Design review of the part built by this model. Coordinates are the model's own, in mm. Face numbers are marked on the shaded views. A direction names the side the tool comes from. Round coordinates to 2 decimals unless told otherwise and drop trailing zeros. Loops run counter-clockwise (first coordinate to the right, second up) from the corner with the lowest first, then second, coordinate; pieces in that order, holes last. Notation, with made-up numbers: (45, -39) - (93, -39) arc R22 cw to (93, -5) - close; hole circle Ø3 at (36.25, -19.5). An arc over 180 degrees is marked (long way). Return JSON: item names as keys, results as strings. Group by question number.
(1) We need section B-B, the plane z = 6.35. Write out the cut boundary in (x, y) (1 decimal), and give its area (3 significant figures).
(2) The part is to be moulded in two halves that separate along Y. For the marked faces 1, 2 and 3, say which applies: pulls with the +Y half, pulls with the -Y half, needs draft (parallel to the pull), parting line crosses it, or undercut.
(3) Clearance check with flat-ended pins moving along their axes: pin 1 (9 mm diameter, centred on x = 26.67, z = 6.35, fed in from -Y) (3 decimals); pin 2 (3 mm diameter, centred on x = 21, y = 0.5, fed in from -Z); pin 3 (10 mm diameter, centred on y = 11, z = 3, fed in from -X); pin 4 (12.5 mm diameter, centred on x = 32.5, y = 11, fed in from +Z). State where each tip first meets the part, or that it passes through.
(4) For the marked faces 4 and 5, list the 3-axis set-ups (+Z, -Z, +X, -X, +Y, -Y) from which the entire face can be reached by the end or side of a thin tool; tool diameter is ignored.
(5) We need section D-D, the plane y = 4.5. Write out the cut boundary in (x, z), and give its area (3 significant figures).
(6) Wall thickness on L1, parallel to X at y = -2.4, z = 6.35; L2, parallel to Y at x = 31, z = 4.5 (1 decimal); L3, parallel to X at y = -5, z = 6.35: over which ranges is each line inside the solid? List them lowest first. Write a range as [from, to].
(7) We need section A-A, the plane x = 26.67. Give the number of separate pieces and of enclosed holes in the cut face, and give its area (3 significant figures).
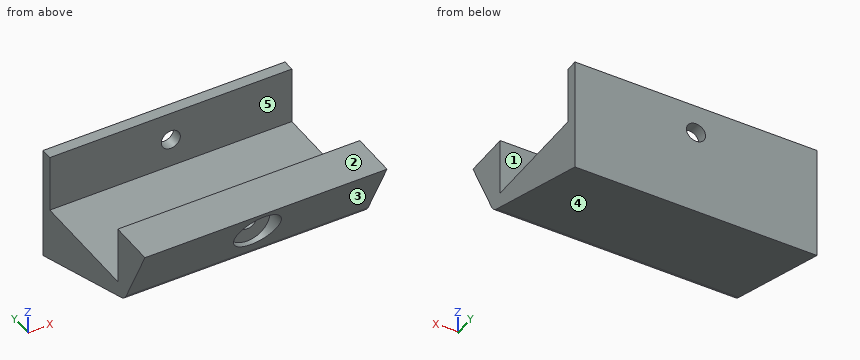
Autodesk Inventor part; units mm, degrees
ref_plane "YZ Plane" through (0, 0, 0) normal (1, 0, 0) x (0, 1, 0)
ref_plane "XZ Plane" through (0, 0, 0) normal (0, 1, 0) x (-1, 0, 0)
ref_plane "XY Plane" through (0, 0, 0) normal (0, 0, 1) x (1, 0, 0)
sketch "Sketch1" plane through (0, 0, 0) normal (1, 0, 0) x (0, 1, 0)
  line L0 (0, 0) -> (25.4, 0)
  line L1 (25.4, 0) -> (25.4, 12.7)
  line L2 (0, 0) -> (0, 12.7)
  line L3 (25.4, 12.7) -> (27.9305, 12.7)
  line L4 (27.9305, 12.7) -> (27.9305, 0)
  line L5 (0, 12.7) -> (-2.54, 12.7)
  line L6 (-2.54, 12.7) -> (-2.54, 0)
  line L7 (-2.54, 0) -> (-2.54, -2.54)
  line L8 (27.9305, -2.54) -> (27.9305, 0)
  line L9 (-2.54, -2.54) -> (-2.54, -12.7002)
  line L10 (27.9305, -12.7002) -> (27.9305, -2.54)
  line L11 (27.9305, -12.7002) -> (-2.54, -2.54)
  line L12 (-2.54, 12.7) -> (-10.16, 12.7)
  line L13 (-10.16, 12.7) -> (-2.54, -2.54)
  line L14 (-2.54, -2.54) -> (0, -2.54)
  dimension "d0" = 25.4
  dimension "d1" = 12.7
  dimension "d2" = 2.54
  dimension "d3" = 2.54
  dimension "d4" = 7.62
extrude "Extrusion1" add sketch "Sketch1" along normal blind 53.34
sketch "Sketch2" plane through (0, 27.9305, 12.7) normal (0, 1, 0) x (1, 0, 0)
  line L0 (0, 0) -> (0, 12.7)
  line L1 (0, 0) -> (0, 6.35)
  line L2 (0, 6.35) -> (26.67, 6.35)
  circle A0 centre (26.67, 6.35) radius 2.1082
  dimension "d7" = 6.35
  dimension "d8" = 26.67
  dimension "d9" = 4.2164
extrude "Extrusion2" cut sketch "Sketch2" against normal blind 54.61
sketch "Sketch3" plane through (0, 0, 0) normal (-1, 0, 0) x (0, 0, 1)
  point P0 (0, 0)
sketch "Sketch4" plane through (0, 0, 12.7) normal (0, 1, 0) x (1, 0, 0)
  circle A0 centre (26.67, 6.35) radius 2.1082
  circle A1 centre (26.67, 6.35) radius 2.1082
  circle A2 centre (26.67, 6.35) radius 5.0752
  point P0 (0, 12.7)
extrude "Extrusion3" cut sketch "Sketch4" against normal up to surface from surface at 0 surface through (0, -10.16, 12.7) normal (0, -0.8944, -0.4472)
sketch "Sketch5" plane through (0, 0, 12.7) normal (0, 1, 0) x (1, 0, 0)
  circle A0 centre (26.67, 6.35) radius 5.0752
  circle A1 centre (26.67, 6.35) radius 5.0752
  circle A2 centre (26.67, 6.35) radius 2.1082
  point P0 (0, 12.7)
  dimension "d14" = 4.2164
extrude "Extrusion4" add sketch "Sketch5" against normal blind 3.175
fillet "Fillet1" radius 3.175 1 edges at (26.67, -2.54, -2.54)
properties part number "sleds v1"
Solutions:
{
 "1": {"outline": "(0, -7) - (21.6, -7) - (21.6, -3.2) - (24.6, -3.2) - (24.6, 0) - (0, 0) - close; (0, 25.4) - (24.6, 25.4) - (24.6, 27.9) - (0, 27.9) - close; (28.8, -3.2) - (31.7, -3.2) - (31.7, -7) - (53.3, -7) - (53.3, 0) - (28.8, 0) - close; (28.8, 25.4) - (53.3, 25.4) - (53.3, 27.9) - (28.8, 27.9) - close", "area": "445 mm^2"},
 "2": {"face 1": "undercut", "face 2": "needs draft", "face 3": "pulls with the -Y half"},
 "3": {"pin 1": "y = -3.175", "pin 2": "z = -4.05", "pin 3": "x = 0", "pin 4": "z = 0"},
 "4": {"face 4": "-Z, +X, -X, -Y", "face 5": "+Z, +X, -X"},
 "5": {"outline": "(0, -4.89) - (53.34, -4.89) - (53.34, 0) - (0, 0) - close", "area": "261 mm^2"},
 "6": {"L1": "[0, 24.56], [28.78, 53.34]", "L2": "[-3.2, 0], [25.4, 27.9]", "L3": "[0, 21.59], [31.75, 53.34]"},
 "7": {"separate pieces": "3", "enclosed holes": "0", "area": "292 mm^2"}
}
